The listing builds one solid part. Answer for the finished solid, in the listing's coordinates (mm). A direction names the side the tool comes from. Round coordinates to 2 decimals unless told otherwise and drop trailing zeros. Write each loop counter-clockwise with the first axis right and the second up, starting at its lowest first coordinate (ties: lowest second). Pieces come first, ordered by that corner, then holes.
Item 1: Find section A-A on y = -12.5. Give the vertices of the cut face in (x, z), then the cut area to 3 significant figures.
Item 2: A tool of negligible diameter and unlimited length cuts with its end or side. For faces 1 (the face through (-117.5, -12.6, 2.5)), 2 (the face through (-15, -12, -5)), 3 (the face through (-10, -15, -10)), from which of +Z, -Z, +X, -X, +Y, -Y can it reach the whole face along a straight path? Write none if from no direction.
Item 3: Find section B-B on z = 2.25. Give the vertices of the cut face in (x, y), then the cut area to 3 significant figures.
Item 4: For a pull along X with two mould halves and no side action, classify faces 4 (the face through (-63, -25, 2)), 5 (the face through (-24.237, -16.33, -4.93)), 6 (the face through (-77, -17.5, 2)) as +X half, -X half, draft (parallel to the pull), parting line (faces both ways), or undercut.
Item 5: Find section C-C on x = -74.5. Give the vertices of the cut face in (y, z), then the cut area to 3 significant figures.
Item 6: Find section D-D on x = -15. Give the vertices of the cut face in (y, z).
Item 7: Find the intervals of material crossed by probe 1 along Y at (x, z) = (-15.5, -8.75); probe 2 along Y at (x, z) = (-110, 1); probe 3 along Z at (x, y) = (-44, -18.75), in increasing order.
Item 8: Each of these flat-tipped pins is pushed along its axis until it touches: pin 1 (1 mm diameter, centred on y = -5, z = -3.5, fed in from +X); pin 2 (12.5 mm diameter, centred on x = -79, y = -7.5, fed in from -Z); pin 3 (5 mm diameter, centred on y = -15.5, z = -7.5, fed in from +X). Where does it stop, or does it pass through?
```python
from build123d import *

# Parameters (mm, degrees)
SKETCH1_W           = 125
SKETCH1_H           = 25
BOSS_EXTRUDE1_DEPTH = 5
SKETCH2_R           = 10
BOSS_EXTRUDE2_DEPTH = 5
SKETCH3_R           = 10
SKETCH3_R_2         = 5
BOSS_EXTRUDE3_DEPTH = 5


with BuildPart() as part:
    # Sketch1 → Boss-Extrude1 (new body)
    with BuildSketch(Plane.XY):
        with Locations((-62.5, -12.5)):
            Rectangle(SKETCH1_W, SKETCH1_H)
        with BuildLine():
            Line((-112.5, -7.5), (-42.5, -7.5))
            ThreePointArc((-42.5, -7.5), (-37.5, -12.5), (-42.5, -17.5))
            Line((-42.5, -17.5), (-112.5, -17.5))
            ThreePointArc((-112.5, -17.5), (-117.5, -12.5), (-112.5, -7.5))
        make_face(mode=Mode.SUBTRACT)
    extrude(amount=BOSS_EXTRUDE1_DEPTH)

    # Sketch2 → Boss-Extrude2 (add)
    with BuildSketch(Plane(origin=(0, 0, 0), x_dir=(-1, 0, 0), z_dir=(0, 0, -1))):
        with Locations((15, -12.5)):
            Circle(SKETCH2_R)
    extrude(amount=BOSS_EXTRUDE2_DEPTH)

    # Sketch3 → Boss-Extrude3 (add)
    with BuildSketch(Plane(origin=(0, 0, -5), x_dir=(-1, 0, 0), z_dir=(0, 0, -1))):
        with Locations((15, -12.5)):
            Circle(SKETCH3_R)
        with Locations((15, -12.5)):
            Circle(SKETCH3_R_2, mode=Mode.SUBTRACT)
    extrude(amount=BOSS_EXTRUDE3_DEPTH)


solid = part.part
```
Check values:
1. outline: (-125, 0) - (-117.5, 0) - (-117.5, 5) - (-125, 5) - close; (-37.5, 0) - (-25, 0) - (-25, -10) - (-20, -10) - (-20, -5) - (-10, -5) - (-10, -10) - (-5, -10) - (-5, 0) - (0, 0) - (0, 5) - (-37.5, 5) - close
1. area: 375 mm2
2. face 1: +Z, -Z
2. face 2: -Z
2. face 3: -Z, +X, -X, +Y, -Y
3. outline: (-125, -25) - (0, -25) - (0, 0) - (-125, 0) - close; hole (-112.5, -17.5) - (-42.5, -17.5) arc R5 ccw to (-42.5, -7.5) - (-112.5, -7.5) arc R5 ccw to start
3. area: 2,350 mm2
4. face 4: draft
4. face 5: parting line
4. face 6: undercut
5. outline: (-25, 0) - (-17.5, 0) - (-17.5, 5) - (-25, 5) - close; (-7.5, 0) - (0, 0) - (0, 5) - (-7.5, 5) - close
5. area: 75.0 mm2
6. outline: (-25, 0) - (-22.5, 0) - (-22.5, -10) - (-17.5, -10) - (-17.5, -5) - (-7.5, -5) - (-7.5, -10) - (-2.5, -10) - (-2.5, 0) - (0, 0) - (0, 5) - (-25, 5) - close
7. probe 1: y = -22.49 to -17.47, -7.53 to -2.51
7. probe 2: y = -25 to -17.5, -7.5 to 0
7. probe 3: z = 0 to 5
8. pin 1: stops at x = -7.86
8. pin 2: stops at z = 0
8. pin 3: stops at x = -5.01
